```python
from build123d import *

# Parameters (mm, degrees)
F0_W     = 20.7
F0_H     = 4
F1_DEPTH = 2
F2_R     = 1.99999
F3_R     = 0.2
F4_R     = 1
F5_DEPTH = 25


# Not quite as in the source:
# - a fillet or chamfer is up to 0.001 mm smaller than in the source, because OpenCascade refuses the exact size


with BuildPart() as f1:
    # F0 (on Front) → F1 (new body)
    with BuildSketch(Plane.XZ):
        with Locations((-0.2598203719, 2.9809341038)):
            Rectangle(F0_W, F0_H)
    extrude(amount=F1_DEPTH)

    # F2 (radius 2 in the source; OpenCascade refuses exactly that, so slightly less here)
    f2_edges = [f1.edges().sort_by_distance(p)[0] for p in [
        (-10.60982, -1, 4.980934),
        (-10.60982, -1, 0.980934),
        (10.09018, -1, 4.980934),
        (10.09018, -1, 0.980934),
    ]]
    fillet(f2_edges, radius=F2_R)

    # F3
    f3_edges = [f1.edges().sort_by_distance(p)[0] for p in [
        (-0.25982, 0, 4.980934),
        (-0.25982, -2, 4.980934),
    ]]
    fillet(f3_edges, radius=F3_R)

    # F4 (on face) → F5 (cut)
    with BuildSketch(Plane(origin=(0, 0, 0), x_dir=(-1, 0, 0), z_dir=(0, 1, 0))):
        with Locations((8.5788203719, 2.9809341038)):
            Circle(F4_R)
        with Locations((-8.0591796281, 2.9809341038)):
            Circle(F4_R)
    extrude(amount=-F5_DEPTH, mode=Mode.SUBTRACT)


solid = f1.part
```
For this review, take the finished solid that the model builds, in its own axes (mm). Round coordinates to 2 decimals unless told otherwise and drop trailing zeros. Use one line per item in the form item = value.
Q1. Clearance check with a flat-ended pin moving along its axis: pin 1 Ø1.6 at (x, z) = (-8.58, 2.98) entering from -Y. State where the tip first meets the part, or that it passes through.
Resolved:
pin_1 = through
Q2. The part is to be moulded in two halves that separate along Z. For faces 1 (the flat face through (0, 0, 3)), 2 (the cylindrical face through (7.105, -0.986, 3.281)), 3 (the cylindrical face through (9.5, -1, 4.4)), say which applies: released by +Z, released by -Z, zero draft, split by the parting line, or undercut.
Resolved:
face_1 = zero draft
face_2 = undercut
face_3 = released by +Z
Q3. To check wall thickness, follow probe 1 along X at (y, z) = (-1.5, 2.9); probe 2 along X at (y, z) = (-1.1, 3.8); probe 3 along Z at (x, y) = (-9, -0.85). State the ranges of each line that lie inside material, in increasing order. Write a range as from..to.
Resolved:
probe_1 = -10.61..-9.58, -7.58..7.06, 9.06..10.09
probe_2 = -10.43..-9.15, -8.01..7.49, 8.63..9.91
probe_3 = 1.02..2.07, 3.89..4.94
Q4. Consider section A-A (y = -0.65). State how many separate pieces and enclosed holes the cut face has, then the cut area to 3 significant figures.
Resolved:
separate_pieces = 1
enclosed_holes = 2
area = 73.1 mm²
